```python
from build123d import *

# Parameters (mm, degrees)
SKETCH1_R           = 2.2225
BOSS_EXTRUDE3_DEPTH = 6.35
CUT_EXTRUDE1_DEPTH  = 6.35
SKETCH3_R           = 2.00025
CUT_EXTRUDE2_DEPTH  = 6.35
SKETCH4_R           = 2.00025
CUT_EXTRUDE3_DEPTH  = 6.35


with BuildPart() as part:
    # Sketch1 → Boss-Extrude3 (new body)
    with BuildSketch(Plane(origin=(0, 0, 0), x_dir=(1, 0, 0), z_dir=(0, 1, 0))):
        Polygon((-6.35, 10.15), (-6.35, 22.85), (-15.08, 22.85), (-27.328680476, 1.634663089), (-22.963680476, -5.925738686), (-11.965157848, 0.424261314), (-5.615157848, -10.574261314), (-16.613680476, -16.924261314), (-12.248680476, -24.484663089), (12.248680476, -24.484663089), (16.613680476, -16.924261314), (5.615157848, -10.574261314), (11.965157848, 0.424261314), (22.963680476, -5.925738686), (27.328680476, 1.634663089), (15.08, 22.85), (6.35, 22.85), (6.35, 10.15), align=None)
        with Locations(Location((0, -20.085254038, 0), (0, 0, 270))):
            Circle(SKETCH1_R, mode=Mode.SUBTRACT)
        with Locations(Location((17.394340238, 10.042627019, 0), (0, 0, 270))):
            Circle(SKETCH1_R, mode=Mode.SUBTRACT)
        with Locations(Location((-17.394340238, 10.042627019, 0), (0, 0, 270))):
            Circle(SKETCH1_R, mode=Mode.SUBTRACT)
        with Locations(Location((0, 0, 0), (0, 0, 270))):
            Circle(SKETCH1_R, mode=Mode.SUBTRACT)
    extrude(amount=BOSS_EXTRUDE3_DEPTH)

    # Sketch2 → Cut-Extrude1 (cut)
    with BuildSketch(Plane(origin=(19.788680476, 0, 11.425), x_dir=(0.5000000000000057, 0, -0.8660254037844354), z_dir=(0.8660254037844354, 0, 0.5000000000000057))):
        with BuildLine():
            ThreePointArc((-11.52525, 3.175), (-9.525, 1.17475), (-7.52475, 3.175))
            Line((-7.52475, 3.175), (-11.52525, 3.175))
        make_face()
        with BuildLine():
            Line((-11.52525, 3.175), (-7.52475, 3.175))
            ThreePointArc((-7.52475, 3.175), (-9.525, 5.17525), (-11.52525, 3.175))
        make_face()
        with BuildLine():
            ThreePointArc((7.52475, 3.175), (9.525, 1.17475), (11.52525, 3.175))
            Line((11.52525, 3.175), (7.52475, 3.175))
        make_face()
        with BuildLine():
            Line((7.52475, 3.175), (11.52525, 3.175))
            ThreePointArc((11.52525, 3.175), (9.525, 5.17525), (7.52475, 3.175))
        make_face()
    extrude(amount=-CUT_EXTRUDE1_DEPTH, mode=Mode.SUBTRACT)

    # Sketch3 → Cut-Extrude2 (cut)
    with BuildSketch(Plane(origin=(-19.788680476, 0, 11.425), x_dir=(0.5000000000000099, 0, 0.866025403784433), z_dir=(-0.8660254037844329, 0, 0.5000000000000098))):
        with Locations((-9.525, 3.175)):
            Circle(SKETCH3_R)
        with Locations((9.525, 3.175)):
            Circle(SKETCH3_R)
    extrude(amount=-CUT_EXTRUDE2_DEPTH, mode=Mode.SUBTRACT)

    # Sketch4 → Cut-Extrude3 (cut)
    with BuildSketch(Plane(origin=(0, 0, -22.85), x_dir=(-1, 0, 0), z_dir=(0, 0, -1))):
        with Locations((-9.525, 3.175)):
            Circle(SKETCH4_R)
        with Locations((9.525, 3.175)):
            Circle(SKETCH4_R)
    extrude(amount=-CUT_EXTRUDE3_DEPTH, mode=Mode.SUBTRACT)


solid = part.part
```
Verification items for the finished model (mm, model axes). A direction names the side the tool comes from. Round coordinates to 2 decimals unless told otherwise and drop trailing zeros. Write each loop counter-clockwise with the first axis right and the second up, starting at its lowest first coordinate (ties: lowest second). Pieces come first, ordered by that corner, then holes. Notation, with made-up numbers: (13, -12.75) - (62, -12.75) arc R24 ccw to (62, 16.25) - close; hole circle Ø4 at (-33, -3). An arc over 180 degrees is marked (long way). Answer as a JSON object with one key per item and string values. Group by question number.
Q1. Thickness scan on line 1 (X direction, y = 3.75, z = -15); line 2 (Z direction, x = -2, y = 0.75); line 3 (X direction, y = 4.25, z = 1). Record the ranges inside material, lowest first.
Q2. Section check B-B, the plane z = -11. Enter the section's corners in (x, y), plus the area to 3 significant figures.
Q3. Section check A-A, the plane x = 0. Enter the section's corners in (y, z), plus the area to 3 significant figures.
Q4. Tool access check on faces 1 (the flat face through (10, 3, -16.5)), 2 (the flat face through (-12, 3, -22.85)), 3 (the flat face through (13.916, 3.131, 21.597)), 4 (the flat face through (0, 3, -10.15)), 5 (the flat face through (17.39, 3.13, 2.71)). Record the directions out of +Z, -Z, +X, -X, +Y, -Y that give a thin tool (end or side, any length) a straight path to the whole face; none if there is none.
Q5. Mould release check, pull along X, two halves, no side actions. Record for faces 6 (the flat face through (9.513, 3.203, 16.523)), 7 (the flat face through (0, 3, 24.485)), 8 (the flat face through (-21.12, 3.13, -12.39)): released by +X, released by -X, zero draft, split by the parting line, or undercut.
Q6. Section check D-D, the plane z = 9. Enter the section's corners in (x, y), plus the area to 3 significant figures.
Q7. Go/stop test with flat-tipped pins: pin 1 Ø2.5 at (x, z) = (0, 0) entering from +Y; pin 2 Ø3 at (y, z) = (0.5, -15.5) entering from -X; pin 3 Ø2 at (x, y) = (18, 5) entering from +Z. Record where each tip stops, or that it passes through.
Q8. Section check C-C, the plane z = -6. Enter the section's corners in (x, y), plus the area to 3 significant figures.
Found:
{
 "1": {"line 1": "x = -19.61 to -6.35, 6.35 to 19.61", "line 2": "z = -10.15 to -0.97, 0.97 to 19.12, 21.05 to 24.48", "line 3": "x = -25.81 to -24.16, -18.48 to -14.43, -11.14 to -1.98, 1.98 to 11.14, 14.43 to 18.48, 24.16 to 25.81"},
 "2": {"outline": "(-21.92, 0) - (-19.4, 0) - (-19.4, 6.35) - (-21.92, 6.35) - close; (-15.39, 0) - (-6.35, 0) - (-6.35, 6.35) - (-15.39, 6.35) - close; (6.35, 0) - (15.39, 0) - (15.39, 6.35) - (6.35, 6.35) - close; (19.4, 0) - (21.92, 0) - (21.92, 6.35) - (19.4, 6.35) - close", "area": "147 mm^2"},
 "3": {"outline": "(0, -10.15) - (6.35, -10.15) - (6.35, -2.22) - (0, -2.22) - close; (0, 2.22) - (6.35, 2.22) - (6.35, 17.86) - (0, 17.86) - close; (0, 22.31) - (6.35, 22.31) - (6.35, 24.48) - (0, 24.48) - close", "area": "163 mm^2"},
 "4": {"face 1": "-Z", "face 2": "-Z, +X, -X, +Y, -Y", "face 3": "+Z, +X, +Y, -Y", "face 4": "-Z, +Y, -Y", "face 5": "+Y, -Y"},
 "5": {"face 6": "undercut", "face 7": "zero draft", "face 8": "released by -X"},
 "6": {"outline": "(-6.52, 0) - (6.52, 0) - (6.52, 6.35) - (-6.52, 6.35) - close", "area": "82.9 mm^2"},
 "7": {"pin 1": "passes through", "pin 2": "stops at x = -20.19", "pin 3": "stops at z = 3.64"},
 "8": {"outline": "(-24.81, 0) - (24.81, 0) - (24.81, 6.35) - (-24.81, 6.35) - close", "area": "315 mm^2"}
}
